from build123d import *

# Parameters (mm, degrees)
BOSS_EXTRUDE1_DEPTH = 19.05


with BuildPart() as part:
    # Sketch1 → Boss-Extrude1 (new body)
    with BuildSketch(Plane.XY):
        with BuildLine():
            Line((152.224173193, 179.795336584), (97.403993572, 735.828587024))
            add(Edge.make_bspline(
                [(0, 803.26908628), (0.979817658, 803.233925105), (2.950075123, 803.151909058), (6.800362849, 802.946009068), (11.504912112, 802.608232022), (16.957304332, 802.075979486), (23.975792063, 801.198424891), (32.273128008, 799.790052384), (41.46699497, 797.614109593), (49.89784204, 794.967332344), (60.129456963, 790.832450746), (71.050790712, 784.572420078), (79.648241417, 776.932392043), (85.274313562, 769.943199813), (88.89525226, 764.228265264), (91.933130485, 758.00316425), (93.979934001, 752.359286407), (95.321414001, 747.554999291), (96.177362738, 743.805316844), (96.764020616, 740.553537606), (97.155379667, 737.881968465), (97.326205951, 736.51096636), (97.403993572, 735.828587024)],
                knots=[0.000508173, 0.000508173, 0.000508173, 0.000508173, 0.016098161, 0.031688149, 0.062868125, 0.094048101, 0.125228077, 0.187588029, 0.249947981, 0.312307933, 0.374667885, 0.499387789, 0.624107693, 0.686467645, 0.748827597, 0.811187549, 0.873547501, 0.904727477, 0.935907453, 0.967087429, 0.982677417, 0.998267405, 0.998267405, 0.998267405, 0.998267405], degree=3))
            add(Edge.make_bspline(
                [(-97.403993572, 735.828587024), (-97.326205951, 736.51096636), (-97.155379667, 737.881968465), (-96.764020616, 740.553537606), (-96.177362738, 743.805316844), (-95.321414001, 747.554999291), (-93.979934001, 752.359286407), (-91.933130485, 758.00316425), (-88.89525226, 764.228265264), (-85.274313562, 769.943199813), (-79.648241417, 776.932392043), (-71.050790712, 784.572420078), (-60.129456963, 790.832450746), (-49.89784204, 794.967332344), (-41.46699497, 797.614109593), (-32.273128008, 799.790052384), (-23.975792063, 801.198424891), (-16.957304332, 802.075979486), (-11.504912112, 802.608232022), (-6.800362849, 802.946009068), (-2.950075123, 803.151909058), (-0.979817658, 803.233925105), (0, 803.26908628)],
                knots=[0.000508173, 0.000508173, 0.000508173, 0.000508173, 0.016098161, 0.031688149, 0.062868125, 0.094048101, 0.125228077, 0.187588029, 0.249947981, 0.312307933, 0.374667885, 0.499387789, 0.624107693, 0.686467645, 0.748827597, 0.811187549, 0.873547501, 0.904727477, 0.935907453, 0.967087429, 0.982677417, 0.998267405, 0.998267405, 0.998267405, 0.998267405], degree=3))
            Line((-97.403993572, 735.828587024), (-102.381323889, 685.344236665))
            Line((-102.381323889, 685.344236665), (-111.860365766, 686.278790089))
            Line((-111.860365766, 686.278790089), (-106.876080835, 736.833680097))
            add(Edge.make_bspline(
                [(-106.876080835, 736.833680097), (-98.655564568, 809.385111394), (0, 812.8)],
                knots=[0, 0, 0, 1, 1, 1], degree=2))
            add(Edge.make_bspline(
                [(106.876080835, 736.833680097), (98.655564568, 809.385111394), (0, 812.8)],
                knots=[0, 0, 0, 1, 1, 1], degree=2))
            Line((106.876080835, 736.833680097), (161.70321507, 180.729890008))
            Line((161.70321507, 180.729890008), (152.224173193, 179.795336584))
        make_face()
    extrude(amount=BOSS_EXTRUDE1_DEPTH)


solid = part.part
Source: CAD feature listing. Evaluate the final solid. Frame: model axes, mm. A direction names the side the tool comes from. Coordinates: 2 decimals unless noted, no trailing zeros. Order: outer loops, then holes, each group sorted by start corner. A loop starts at its lowest first (then second) coordinate and runs counter-clockwise, first axis right, second up.
Item 1: Set-up query: faces 1 (the face through (-99.858, 710.94, 9.392)), 2 (the face through (117, 592, 19.05)). Return all of +Z, -Z, +X, -X, +Y, -Y with unobstructed straight access to the full face (end or side cutting, diameter ignored); none if empty.
Output values:
face 1: +Z, -Z, -Y
face 2: +Z, +X, -X, +Y, -Y
Item 2: Material intervals for line 1 (X direction, y = 708, z = 13.25); line 2 (X direction, y = 735, z = 7.5); line 3 (Y direction, x = 68.5, z = 12.5), sorted ascending.
Output values:
line 1: x = -109.72 to -100.15, 100.15 to 109.72
line 2: x = -107.06 to -97.49, 97.49 to 107.06
line 3: y = 785.73 to 796.87
Item 3: First-contact query: P1, Ø1.5, axis at y = 641, z = 3.5, coming from the +X side; P2, Ø1.5, axis at y = 453.5, z = 12.5, coming from the -X side; P3, Ø4, axis at x = 22.5, z = 2, coming from the +Y side; P4, Ø3, axis at x = 109, y = 679.5, coming from the -Z side. Flat tips, straight axial feed; report the tip coordinate or a pass-through.
Output values:
P1: stops at x = 116.4
P2: stops at x = 125.17
P3: stops at y = 811.23
P4: stops at z = 0
Item 4: Cut plane A-A (y = 594). Return loops of the section in (x, z), plus the area to 3 significant figures.
Output values:
outline: (111.39, 0) - (120.96, 0) - (120.96, 19.05) - (111.39, 19.05) - close
area: 182 mm2
